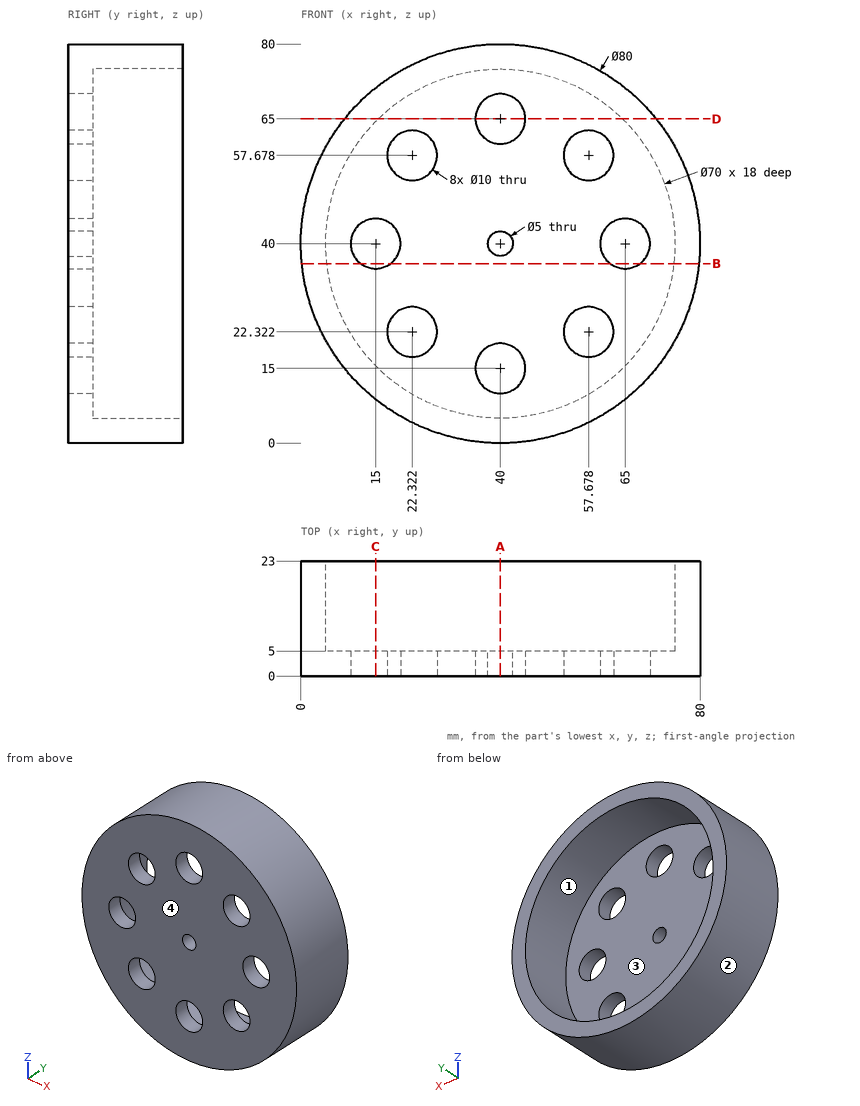
Job drawing, mm, ordinate dimensions from the low corner. One solid piece. Give positions to 0.01 mm unless a question says otherwise; leave off trailing zeros. Loops run counter-clockwise (first coordinate to the right, second up) from the corner with the lowest first, then second, coordinate; pieces in that order, holes last. Notation, with made-up numbers: M 31,76.25 L 42,76.25 A14 ccw 42,102.25 Z; hole C -23.5,87 d4. An arc over 180 degrees is marked long. Put each result on its own line as item: value. Start each with the question number.
1) Saw through at D-D (z = 65). List the corners of the cut face in (x, y) (1 decimal).
2) Saw through at A-A (x = 40). List the corners of the cut face in (y, z).
3) Saw through at C-C (x = 15). List the corners of the cut face in (y, z) (1 decimal).
4) Flat gauge pins, fed straight in: pin 1 (5 mm diameter, centred on x = 35.5, y = 11, fed in from -Z); pin 2 (1 mm diameter, centred on x = 57.5, y = 14, fed in from +Z); pin 3 (6 mm diameter, centred on x = 10.5, y = 20.5, fed in from +Z). Where does each tip first touch, or does it go through?
5) Saw through at B-B (z = 36). List the corners of the cut face in (x, y), then the cut area to 3 significant figures.
6) Probe probe 1 along X at (y, z) = (3.3, 40); probe 2 along X at (y, z) = (14.5, 40); probe 3 along Y at (x, z) = (55.5, 64). List the from-to ranges inside material, lowest first.
7) Pull direction Z, two halves, no side cores. Call the marked faces 1, 2, 3 and 4: +Z half, -Z half, draft (parallel to the pull), parting line (faces both ways), or undercut.
Numbers:
1. outline: M 8.8,0 L 35,0 L 35,5 L 15.5,5 L 15.5,23 L 8.8,23 Z; M 45,0 L 71.2,0 L 71.2,23 L 64.5,23 L 64.5,5 L 45,5 Z
2. outline: M 0,0 L 23,0 L 23,5 L 5,5 L 5,10 L 0,10 Z; M 0,20 L 5,20 L 5,37.5 L 0,37.5 Z; M 0,42.5 L 5,42.5 L 5,60 L 0,60 Z; M 0,70 L 5,70 L 5,75 L 23,75 L 23,80 L 0,80 Z
3. outline: M 0,8.8 L 23,8.8 L 23,15.5 L 5,15.5 L 5,35 L 0,35 Z; M 0,45 L 5,45 L 5,64.5 L 23,64.5 L 23,71.2 L 0,71.2 Z
4. pin 1: z = 0.05
4. pin 2: z = 76.21
4. pin 3: z = 69.96
5. outline: M 0.2,0 L 12,0 L 12,5 L 5.23,5 L 5.23,23 L 0.2,23 Z; M 18,0 L 62,0 L 62,5 L 18,5 Z; M 68,0 L 79.8,0 L 79.8,23 L 74.77,23 L 74.77,5 L 68,5 Z
5. area: 519 mm^2
6. probe 1: 0 to 10, 20 to 37.5, 42.5 to 60, 70 to 80
6. probe 2: 0 to 5, 75 to 80
6. probe 3: 0 to 5
7. face 1: undercut
7. face 2: parting line
7. face 3: undercut
7. face 4: draft
